Source: CAD feature listing. Evaluate the final solid. Frame: model axes, mm. A direction names the side the tool comes from. Round coordinates to 2 decimals unless told otherwise and drop trailing zeros. Order: outer loops, then holes, each group sorted by start corner. A loop starts at its lowest first (then second) coordinate and runs counter-clockwise, first axis right, second up. Notation, with made-up numbers: (51, -29.75) - (94, -29.75) arc R6 cw to (94, -20.75) - close; hole circle Ø9 at (-5.5, 37). An arc over 180 degrees is marked (long way). Put each result on its own line as item: value. Start each with the question number.
1) Section A-A on x = 40. Output: boundary loops of the cut face in (y, z), then the cut area to 3 significant figures.
2) Contact query for flat-ended pins moving along their axis: P1, Ø0.9, axis at y = -24.5, z = -9, coming from the -X side; P2, Ø2.5, axis at y = 25.5, z = -9.5, coming from the +X side; P3, Ø0.9, axis at y = 0, z = 1, coming from the -X side; P4, Ø2, axis at y = 17.5, z = -2, coming from the +X side. Output: stop coordinate, or through.
3) Access query for faces 1 (the face through (59.388, 0, 1)), 2 (the face through (39, 3.911, 1)), 3 (the face through (-20.612, 25, -6)), 4 (the face through (-16, -22.479, -6)), 5 (the face through (-10.612, 25, -6)). Directions: +Z, -Z, +X, -X, +Y, -Y. A direction counts if a zero-diameter tool reaches every point of the face in a straight line with its end or side. Return the directions, or none.
4) Mould query, pull axis X, two halves, no side actions, for faces 6 (the face through (-45.612, 1, 1)), 7 (the face through (-10.612, -24, -6)), 8 (the face through (-16, 25, -13)), 9 (the face through (11, 6.817, 1)). Classes: +X half, -X half, draft (parallel to the pull), parting line (faces both ways), or undercut.
5) Section C-C on y = 0.5. Output: boundary loops of the cut face in (x, z).
6) Section D-D on z = 2. Output: boundary loops of the cut face in (x, y).
7) Line query: probe 1 along Y at (x, z) = (45, 0.5); probe 2 along Y at (x, z) = (39.5, -1.75); probe 3 along X at (y, z) = (-4, 1.75). Output: solid intervals per line, ascending. Write a range as [from, to].
8) Section B-B on z = -4. Output: boundary loops of the cut face in (x, y).
```python
from build123d import *

# Parameters (mm, degrees)
SKETCH_W     = 107
SKETCH_H     = 52
SKETCH_W_2   = 19
SKETCH_H_2   = 18.075611
SKETCH_W_3   = 26
SKETCH_H_3   = 15
PAD_DEPTH    = 3
FILLET_R     = 1
SKETCH001_W  = 1
SKETCH001_H  = 7
POCKET_DEPTH = 3.001
SKETCH002_W  = 10
SKETCH002_H  = 3
PAD001_DEPTH = 13


with BuildPart() as part:
    # Sketch → Pad (new body)
    with BuildSketch(Plane.XY):
        with Locations((6.888296, 0.52123)):
            Rectangle(SKETCH_W, SKETCH_H)
        with Locations((11.388296, -2.220965)):
            Rectangle(SKETCH_W_2, SKETCH_H_2, mode=Mode.SUBTRACT)
        with Locations((39.388296, -3.58877)):
            Rectangle(SKETCH_W_3, SKETCH_H_3, mode=Mode.SUBTRACT)
    extrude(amount=PAD_DEPTH)

    # Fillet
    fillet_edges = [part.edges().sort_by_distance(p)[0] for p in [
        (-46.611704, 26.52123, 1.5),
        (60.388296, 26.52123, 1.5),
        (60.388296, -25.47877, 1.5),
        (-46.611704, -25.47877, 1.5),
    ]]
    fillet(fillet_edges, radius=FILLET_R)

    # Sketch001 (on ShapeBinder) → Pocket (cut, through all)
    with BuildSketch(Plane(origin=(0, 0, 0), x_dir=(1, 0, 0), z_dir=(0, 0, -1))):
        with Locations((-46.111704, -0.481376)):
            Rectangle(SKETCH001_W, SKETCH001_H)
        with Locations((59.888296, 0)):
            Rectangle(SKETCH001_W, SKETCH001_H)
    extrude(amount=-POCKET_DEPTH, mode=Mode.SUBTRACT)

    # Sketch002 (on ShapeBinder) → Pad001 (join)
    with BuildSketch(Plane(origin=(0, 0, 0), x_dir=(1, 0, 0), z_dir=(0, 0, -1))):
        with Locations((-15.611704, 23.97877)):
            Rectangle(SKETCH002_W, SKETCH002_H)
        with Locations((42.388296, 23.97877)):
            Rectangle(SKETCH002_W, SKETCH002_H)
        with Locations((-15.611704, -25.02123)):
            Rectangle(SKETCH002_W, SKETCH002_H)
        with Locations((42.388296, -25.02123)):
            Rectangle(SKETCH002_W, SKETCH002_H)
    extrude(amount=PAD001_DEPTH)


solid = part.part
```
Answer sheet:
1. outline: (-25.48, -13) - (-22.48, -13) - (-22.48, 0) - (-11.09, 0) - (-11.09, 3) - (-25.48, 3) - close; (3.91, 0) - (23.52, 0) - (23.52, -13) - (26.52, -13) - (26.52, 3) - (3.91, 3) - close
1. area: 189 mm^2
2. P1: x = -20.61
2. P2: x = 47.39
2. P3: x = -45.61
2. P4: through
3. face 1: +Z, -Z, +X
3. face 2: +Z, -Z
3. face 3: -Z, -X, +Y, -Y
3. face 4: -Z, +X, -X
3. face 5: -Z, +Y, -Y
4. face 6: -X half
4. face 7: undercut
4. face 8: draft
4. face 9: undercut
5. outline: (-45.61, 0) - (1.89, 0) - (1.89, 3) - (-45.61, 3) - close; (20.89, 0) - (26.39, 0) - (26.39, 3) - (20.89, 3) - close; (52.39, 0) - (59.39, 0) - (59.39, 3) - (52.39, 3) - close
6. outline: (-46.61, -24.48) arc R1 ccw to (-45.61, -25.48) - (59.39, -25.48) arc R1 ccw to (60.39, -24.48) - (60.39, -3.5) - (59.39, -3.5) - (59.39, 3.5) - (60.39, 3.5) - (60.39, 25.52) arc R1 ccw to (59.39, 26.52) - (-45.61, 26.52) arc R1 ccw to (-46.61, 25.52) - (-46.61, 3.98) - (-45.61, 3.98) - (-45.61, -3.02) - (-46.61, -3.02) - close; hole (1.89, -11.26) - (20.89, -11.26) - (20.89, 6.82) - (1.89, 6.82) - close; hole (26.39, -11.09) - (52.39, -11.09) - (52.39, 3.91) - (26.39, 3.91) - close
7. probe 1: [-25.48, -11.09], [3.91, 26.52]
7. probe 2: [-25.48, -22.48], [23.52, 26.52]
7. probe 3: [-46.61, 1.89], [20.89, 26.39], [52.39, 60.39]
8. outline: (-20.61, -25.48) - (-10.61, -25.48) - (-10.61, -22.48) - (-20.61, -22.48) - close; (-20.61, 23.52) - (-10.61, 23.52) - (-10.61, 26.52) - (-20.61, 26.52) - close; (37.39, -25.48) - (47.39, -25.48) - (47.39, -22.48) - (37.39, -22.48) - close; (37.39, 23.52) - (47.39, 23.52) - (47.39, 26.52) - (37.39, 26.52) - close
